Verification items for the finished model (mm, model axes). Face numbers are marked on the shaded views. A direction names the side the tool comes from. Round coordinates to 2 decimals unless told otherwise and drop trailing zeros. Order: outer loops, then holes, each group sorted by start corner. A loop starts at its lowest first (then second) coordinate and runs counter-clockwise, first axis right, second up. Notation, with made-up numbers: M 28.25,44 L 32.25,44 A27 cw 32.25,62 Z; hole C 5.25,57.5 d1. An arc over 180 degrees is marked long. One line per item, written item: value. Start each with the question number.
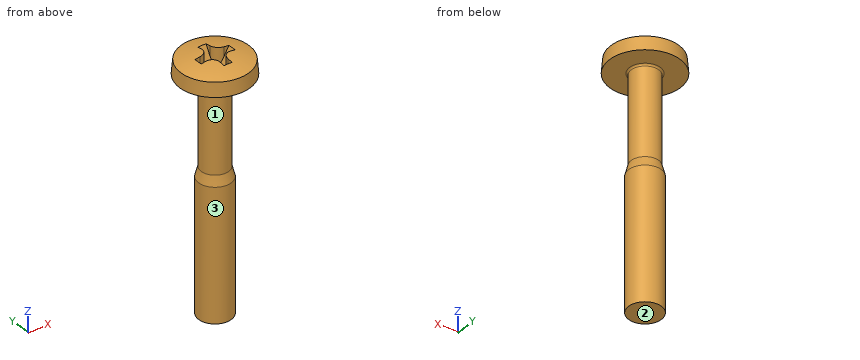
Autodesk Fusion 360 part; units mm, degrees
sketch "Sketch1" plane through (0, 0, 0) normal (0, 1, 0) x (1, 0, 0)
  line L0 (0, -1.2) -> (0, 6)
  line L1 (-2.15, 0) -> (-2.0756, -0.85)
  line L2 (-2.15, 0) -> (-0.8392, 0)
  arc A0 (-2.0756, -0.85) -> (0, -1.2) centre (0, 5.1297) ccw
  line L3 (0, 6) -> (-1, 6)
  line L4 (-1, 6) -> (-1, 0.75)
  line L5 (-1, 0.75) -> (-0.8392, 0.15)
  line L6 (-0.8392, 0.15) -> (-0.8392, 0)
  dimension "d13" = 5
  dimension "d14" = 4.3
  dimension "d18" = 2
  dimension "d23" = 15
  dimension "d53" = 1.2
  dimension "d55" = 5.25
  dimension "d56" = 6
  dimension "d57" = 5.85
  dimension "d60" = 0.85
revolve "Revolve1" add sketch "Sketch1" angle 360 about axis through (0, 0, 1.2) along (0, 0, -1) makes body 1
fillet "Fillet2" radius 0.1 1 edges at (-0.7824, 0.3035, 0) on bodies 1
ref_plane "WorkPlane1" through (0, 0, 1.2) normal (0, 0, 1) x (1, 0, 0)
sketch "Sketch2" plane through (0, 0, 1.2) normal (0, 0, 1) x (1, 0, 0)
  line L0 (-0.248, 0.248) -> (-1.1, 0.248)
  line L1 (-1.1, 0.248) -> (-1.1, -0.248)
  line L2 (-1.1, -0.248) -> (-0.248, -0.248)
  line L3 (-0.248, -0.248) -> (-0.248, -1.1)
  line L4 (-0.248, -1.1) -> (0.248, -1.1)
  line L5 (0.248, -1.1) -> (0.248, -0.248)
  line L6 (0.248, -0.248) -> (1.1, -0.248)
  line L7 (1.1, -0.248) -> (1.1, 0.248)
  line L8 (1.1, 0.248) -> (0.248, 0.248)
  line L9 (0.248, 0.248) -> (0.248, 1.1)
  line L10 (0.248, 1.1) -> (-0.248, 1.1)
  line L11 (-0.248, 1.1) -> (-0.248, 0.248)
  dimension "d63" = 0.496
  dimension "d65" = 360
  dimension "d66" = 2.2
extrude "Extrude1" add sketch "Sketch2" against normal blind 1.01 separate body makes body 2
draft "Draft1" angle -30 neutral plane through (0, 0, 1.2) pull (0, 0, 1) 4 faces at (-0.0827, -1.1, 0.8633) (1.1, -0.0827, 0.8633) (0.0827, 1.1, 0.8633) (-1.1, 0.0827, 0.8633) on bodies 2
fillet "Fillet1" radius 0.496 4 edges at (0.248, -0.248, 0.695) (0.248, 0.248, 0.695) (-0.248, -0.248, 0.695) (-0.248, 0.248, 0.695) on bodies 2
combine "Combine1" operation cut target body 1 tool bodies 2
thread "Thread1" thread offset 0 thread length 10
equation "adsk_nomdia = 2.00 mm"
equation "adsk_nomlen = 6.00 mm"
equation "adsk_headdia = 4.30 mm"
equation "adsk_baseh = 0.85 mm"
equation "adsk_phildia = 2.20 mm"
equation "adsk_midfillet = 0.10 mm"
equation "adsk_thrlen = 5.25 mm"
equation "adsk_phildepth = 1.01 mm"
equation "adsk_thrrun = 0.60 mm"
equation "adsk_thrang = 15.00 deg"
equation "adsk_headang = 5.00 deg"
equation "d13 = adsk_headang"
equation "d14 = adsk_headdia"
equation "adsk_ovalh = 0.35 mm"
equation "d18 = adsk_nomdia"
equation "d23 = adsk_thrang"
equation "d32 = adsk_baseh + adsk_ovalh"
equation "adsk_philwidth = 0.496 mm"
equation "d52 = adsk_midfillet"
equation "d53 = adsk_baseh + adsk_ovalh"
equation "d55 = adsk_thrlen"
equation "d56 = adsk_nomlen"
equation "d57 = adsk_thrlen + adsk_thrrun"
equation "d60 = adsk_baseh"
equation "d63 = adsk_philwidth"
equation "d66 = adsk_phildia"
equation "d68 = adsk_philwidth"
properties part number "BHS JIS B 1111 - M2x6 Acero 4.6 Normal"

Autodesk Fusion 360 part; units mm, degrees
sketch "Sketch1" plane through (0, 0, 0) normal (0, 1, 0) x (1, 0, 0)
  line L0 (0, -1.2) -> (0, 10)
  line L1 (-2.15, 0) -> (-2.0756, -0.85)
  line L2 (-2.15, 0) -> (-0.8392, 0)
  arc A0 (-2.0756, -0.85) -> (0, -1.2) centre (0, 5.1297) ccw
  line L3 (0, 10) -> (-1, 10)
  line L4 (-1, 10) -> (-1, 2)
  line L5 (-1, 2) -> (-0.8392, 1.4)
  line L6 (-0.8392, 1.4) -> (-0.8392, 0)
  dimension "d13" = 5
  dimension "d14" = 4.3
  dimension "d18" = 2
  dimension "d23" = 15
  dimension "d53" = 1.2
  dimension "d55" = 8
  dimension "d56" = 10
  dimension "d57" = 8.6
  dimension "d60" = 0.85
revolve "Revolve1" add sketch "Sketch1" angle 360 about axis through (0, 0, 1.2) along (0, 0, -1) makes body 1
fillet "Fillet2" radius 0.1 1 edges at (-0.7824, 0.3035, 0) on bodies 1
ref_plane "WorkPlane1" through (0, 0, 1.2) normal (0, 0, 1) x (1, 0, 0)
sketch "Sketch2" plane through (0, 0, 1.2) normal (0, 0, 1) x (1, 0, 0)
  line L0 (-0.248, 0.248) -> (-1.1, 0.248)
  line L1 (-1.1, 0.248) -> (-1.1, -0.248)
  line L2 (-1.1, -0.248) -> (-0.248, -0.248)
  line L3 (-0.248, -0.248) -> (-0.248, -1.1)
  line L4 (-0.248, -1.1) -> (0.248, -1.1)
  line L5 (0.248, -1.1) -> (0.248, -0.248)
  line L6 (0.248, -0.248) -> (1.1, -0.248)
  line L7 (1.1, -0.248) -> (1.1, 0.248)
  line L8 (1.1, 0.248) -> (0.248, 0.248)
  line L9 (0.248, 0.248) -> (0.248, 1.1)
  line L10 (0.248, 1.1) -> (-0.248, 1.1)
  line L11 (-0.248, 1.1) -> (-0.248, 0.248)
  dimension "d63" = 0.496
  dimension "d65" = 360
  dimension "d66" = 2.2
extrude "Extrude1" add sketch "Sketch2" against normal blind 1.01 separate body makes body 2
draft "Draft1" angle -30 neutral plane through (0, 0, 1.2) pull (0, 0, 1) 4 faces at (-0.0827, -1.1, 0.8633) (1.1, -0.0827, 0.8633) (0.0827, 1.1, 0.8633) (-1.1, 0.0827, 0.8633) on bodies 2
fillet "Fillet1" radius 0.496 4 edges at (0.248, -0.248, 0.695) (0.248, 0.248, 0.695) (-0.248, -0.248, 0.695) (-0.248, 0.248, 0.695) on bodies 2
combine "Combine1" operation cut target body 1 tool bodies 2
thread "Thread1" thread offset 0 thread length 10
equation "adsk_nomdia = 2.00 mm"
equation "adsk_nomlen = 10.00 mm"
equation "adsk_headdia = 4.30 mm"
equation "adsk_baseh = 0.85 mm"
equation "adsk_phildia = 2.20 mm"
equation "adsk_midfillet = 0.10 mm"
equation "adsk_thrlen = 8.00 mm"
equation "adsk_phildepth = 1.01 mm"
equation "adsk_thrrun = 0.60 mm"
equation "adsk_thrang = 15.00 deg"
equation "adsk_headang = 5.00 deg"
equation "d13 = adsk_headang"
equation "d14 = adsk_headdia"
equation "adsk_ovalh = 0.35 mm"
equation "d18 = adsk_nomdia"
equation "d23 = adsk_thrang"
equation "d32 = adsk_baseh + adsk_ovalh"
equation "adsk_philwidth = 0.496 mm"
equation "d52 = adsk_midfillet"
equation "d53 = adsk_baseh + adsk_ovalh"
equation "d55 = adsk_thrlen"
equation "d56 = adsk_nomlen"
equation "d57 = adsk_thrlen + adsk_thrrun"
equation "d60 = adsk_baseh"
equation "d63 = adsk_philwidth"
equation "d66 = adsk_phildia"
equation "d68 = adsk_philwidth"
properties part number "BHS JIS B 1111 - M2x10 Acero 4.6 Normal"

Autodesk Fusion 360 part; units mm, degrees
sketch "Sketch1" plane through (0, 0, 0) normal (0, 1, 0) x (1, 0, 0)
  line L0 (0, -1.2) -> (0, 14)
  line L1 (-2.15, 0) -> (-2.0756, -0.85)
  line L2 (-2.15, 0) -> (-0.8392, 0)
  arc A0 (-2.0756, -0.85) -> (0, -1.2) centre (0, 5.1297) ccw
  line L3 (0, 14) -> (-1, 14)
  line L4 (-1, 14) -> (-1, 6)
  line L5 (-1, 6) -> (-0.8392, 5.4)
  line L6 (-0.8392, 5.4) -> (-0.8392, 0)
  dimension "d13" = 5
  dimension "d14" = 4.3
  dimension "d18" = 2
  dimension "d23" = 15
  dimension "d53" = 1.2
  dimension "d55" = 8
  dimension "d56" = 14
  dimension "d57" = 8.6
  dimension "d60" = 0.85
revolve "Revolve1" add sketch "Sketch1" angle 360 about axis through (0, 0, 1.2) along (0, 0, -1) makes body 1
fillet "Fillet2" radius 0.1 1 edges at (-0.7824, 0.3035, 0) on bodies 1
ref_plane "WorkPlane1" through (0, 0, 1.2) normal (0, 0, 1) x (1, 0, 0)
sketch "Sketch2" plane through (0, 0, 1.2) normal (0, 0, 1) x (1, 0, 0)
  line L0 (-0.248, 0.248) -> (-1.1, 0.248)
  line L1 (-1.1, 0.248) -> (-1.1, -0.248)
  line L2 (-1.1, -0.248) -> (-0.248, -0.248)
  line L3 (-0.248, -0.248) -> (-0.248, -1.1)
  line L4 (-0.248, -1.1) -> (0.248, -1.1)
  line L5 (0.248, -1.1) -> (0.248, -0.248)
  line L6 (0.248, -0.248) -> (1.1, -0.248)
  line L7 (1.1, -0.248) -> (1.1, 0.248)
  line L8 (1.1, 0.248) -> (0.248, 0.248)
  line L9 (0.248, 0.248) -> (0.248, 1.1)
  line L10 (0.248, 1.1) -> (-0.248, 1.1)
  line L11 (-0.248, 1.1) -> (-0.248, 0.248)
  dimension "d63" = 0.496
  dimension "d65" = 360
  dimension "d66" = 2.2
extrude "Extrude1" add sketch "Sketch2" against normal blind 1.01 separate body makes body 2
draft "Draft1" angle -30 neutral plane through (0, 0, 1.2) pull (0, 0, 1) 4 faces at (-0.0827, -1.1, 0.8633) (1.1, -0.0827, 0.8633) (0.0827, 1.1, 0.8633) (-1.1, 0.0827, 0.8633) on bodies 2
fillet "Fillet1" radius 0.496 4 edges at (0.248, -0.248, 0.695) (0.248, 0.248, 0.695) (-0.248, -0.248, 0.695) (-0.248, 0.248, 0.695) on bodies 2
combine "Combine1" operation cut target body 1 tool bodies 2
thread "Thread1" thread offset 0 thread length 10
equation "adsk_nomdia = 2.00 mm"
equation "adsk_nomlen = 14.00 mm"
equation "adsk_headdia = 4.30 mm"
equation "adsk_baseh = 0.85 mm"
equation "adsk_phildia = 2.20 mm"
equation "adsk_midfillet = 0.10 mm"
equation "adsk_thrlen = 8.00 mm"
equation "adsk_phildepth = 1.01 mm"
equation "adsk_thrrun = 0.60 mm"
equation "adsk_thrang = 15.00 deg"
equation "adsk_headang = 5.00 deg"
equation "d13 = adsk_headang"
equation "d14 = adsk_headdia"
equation "adsk_ovalh = 0.35 mm"
equation "d18 = adsk_nomdia"
equation "d23 = adsk_thrang"
equation "d32 = adsk_baseh + adsk_ovalh"
equation "adsk_philwidth = 0.496 mm"
equation "d52 = adsk_midfillet"
equation "d53 = adsk_baseh + adsk_ovalh"
equation "d55 = adsk_thrlen"
equation "d56 = adsk_nomlen"
equation "d57 = adsk_thrlen + adsk_thrrun"
equation "d60 = adsk_baseh"
equation "d63 = adsk_philwidth"
equation "d66 = adsk_phildia"
equation "d68 = adsk_philwidth"
properties part number "BHS JIS B 1111 - M2x14 Acero 4.6 Normal"
1. Section check B-B (z = -7.5). Record the cut outline in (x, y), and give its area (3 significant figures).
2. Depth check by flat-ended pin: pin 1 (0.8 mm diameter, centred on x = 0, y = 0, fed in from +Z); pin 2 (2 mm diameter, centred on y = -1.5, z = -7.5, fed in from -X); pin 3 (1 mm diameter, centred on y = 0.5, z = -12, fed in from +X). Enter the tip coordinate at first touch or a pass-through.
3. Tool access check on the marked faces 1, 2 and 3. Record the directions out of +Z, -Z, +X, -X, +Y, -Y that give a thin tool (end or side, any length) a straight path to the whole face; none if there is none.
4. Section check A-A (z = -2.75). Record the cut outline in (x, y), and give its area (3 significant figures).
5. Scan lines: line 1 along Z through (x, y) = (0.55, 0.2); line 2 along Z through (x, y) = (0.2, -1.4); line 3 along Y through (x, z) = (-0.3, -8.25). Record each from-to range of solid material in increasing order.
Geometry check:
1. outline: C 0,0 d2
1. area: 3.14 mm²
2. pin 1: stops at z = 0.19
2. pin 2: stops at x = -0.87
2. pin 3: stops at x = 1
3. face 1: none
3. face 2: -Z, +X, -X, +Y, -Y
3. face 3: -Z
4. outline: C 0,0 d1.68
4. area: 2.21 mm²
5. line 1: z = -14 to 0.25
5. line 2: z = 0 to 1.04
5. line 3: y = -0.95 to 0.95
